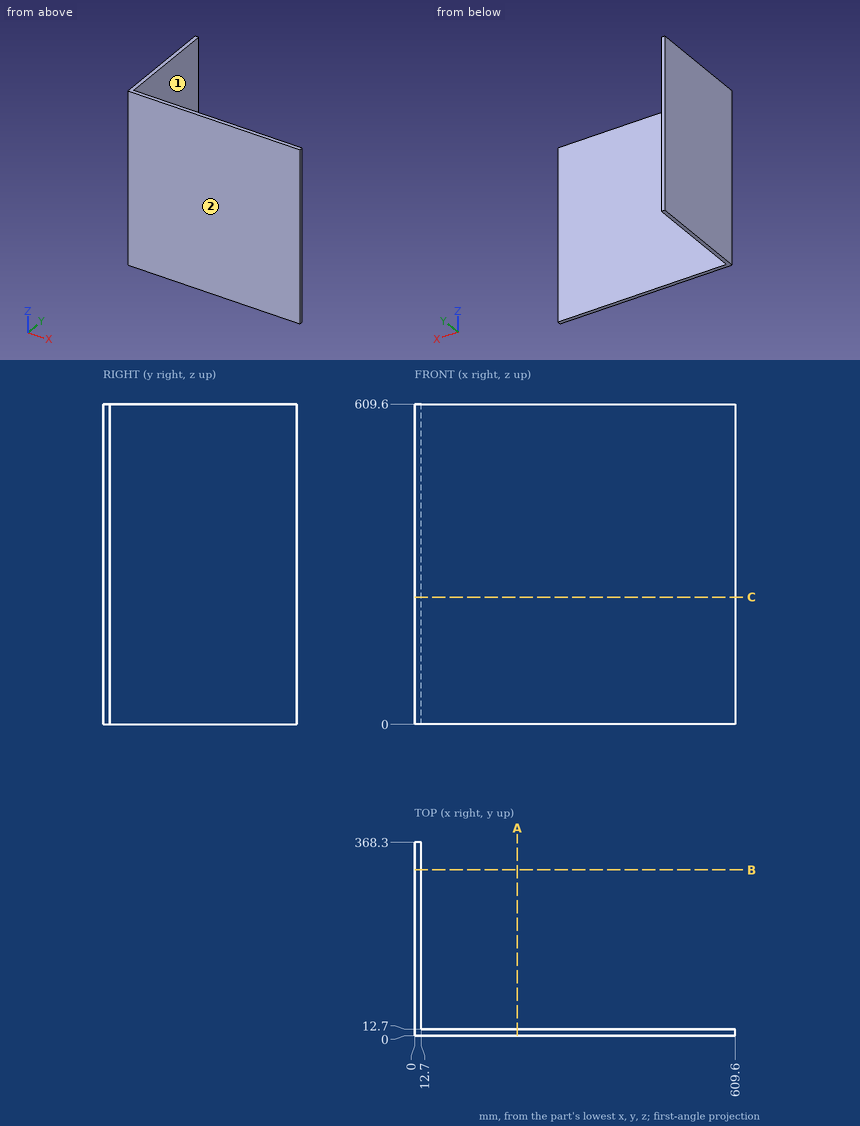
Geometry check sheet. Reference: drawing and pictorial views, mm from the part's lowest x, y, z. A direction names the side the tool comes from. Give positions to 0.01 mm unless a question says otherwise; leave off trailing zeros. Order: outer loops, then holes, each group sorted by start corner. A loop starts at its lowest first (then second) coordinate and runs counter-clockwise, first axis right, second up. Notation, with made-up numbers: M 38,80 L 83,80 A10 cw 83,87 Z; hole C 12,60 d2. An arc over 180 degrees is marked long. Answer in a Markdown table with one row per item. Add a question column.
Q1. Sectioned sample at A-A, the plane x = 195.5. Record the boundary of the cut face in (y, z), and give its area (3 significant figures).
Q2. Gauge pin test, flat ends, axial feed: pin 1 Ø5 at (y, z) = (211.5, 546) entering from -X; pin 2 Ø2 at (x, z) = (165, 276) entering from +Y. Record the tip position at first contact, or that the pin passes through.
Q3. Access from +Z, -Z, +X, -X, +Y, -Y to the whole of each face (thin tool, end or side, straight path). Record for the marked faces 1 and 2.
Q4. Thickness scan on L1, parallel to X at y = 218.5, z = 121. Record the ranges inside material, lowest first.
Q5. Sectioned sample at C-C, the plane z = 242. Record the boundary of the cut face in (x, y), and give its area (3 significant figures).
Verdict:
| question | item | result |
|---|---|---|
| 1 | outline | M 0,0 L 12.7,0 L 12.7,609.6 L 0,609.6 Z |
| 1 | area | 7,740 mm² |
| 2 | pin 1 | x = 0 |
| 2 | pin 2 | y = 12.7 |
| 3 | face 1 | +Z, -Z, +X, +Y |
| 3 | face 2 | +Z, -Z, +X, -X, -Y |
| 4 | L1 | 0 to 12.7 |
| 5 | outline | M 0,0 L 609.6,0 L 609.6,12.7 L 12.7,12.7 L 12.7,368.3 L 0,368.3 Z |
| 5 | area | 12,300 mm² |
